Here's how the part is built. I have some questions about the finished solid (model axes, mm). Face numbers are marked on the shaded views. Round coordinates to 2 decimals unless told otherwise and drop trailing zeros. Order: outer loops, then holes, each group sorted by start corner. A loop starts at its lowest first (then second) coordinate and runs counter-clockwise, first axis right, second up.
```python
from build123d import *

# Parameters (mm, degrees)
CUT_EXTRUDE1_DEPTH      = 13.00023
CUT_EXTRUDE1_DEPTH_BACK = 13.00023
SKETCH3_R               = 7.9375
CUT_EXTRUDE3_DEPTH      = 13.7


with BuildPart() as part:
    # Sketch1 → Revolve1 (revolve)
    with BuildSketch(Plane(origin=(0, 0, 0), x_dir=(1, 0, 0), z_dir=(0, 1, 0))):
        with BuildLine():
            Line((0, 12.00023), (0, -12.00023))
            ThreePointArc((0, -12.00023), (12.00023, 0), (0, 12.00023))
        make_face()
    revolve(axis=Axis((0, 0, -16.515997735), (0, 0, 1)))

    # Sketch2 → Cut-Extrude1 (cut, two sides)
    with BuildSketch(Plane(origin=(0, 0, 0), x_dir=(0, 0, -1), z_dir=(1, 0, 0))) as cut_extrude1_sk:
        with BuildLine():
            Line((-6.35, 10.182485947), (-6.35, -10.182485947))
            ThreePointArc((-6.35, -10.182485947), (-12.00023, 0), (-6.35, 10.182485947))
        make_face()
        with BuildLine():
            ThreePointArc((6.35, -10.182485947), (12.00023, 0), (6.35, 10.182485947))
            Line((6.35, 10.182485947), (6.35, -10.182485947))
        make_face()
    extrude(amount=CUT_EXTRUDE1_DEPTH, mode=Mode.SUBTRACT)
    extrude(cut_extrude1_sk.sketch, amount=-CUT_EXTRUDE1_DEPTH_BACK, mode=Mode.SUBTRACT)

    # Sketch3 → Cut-Extrude3 (cut, through all)
    with BuildSketch(Plane.XY.offset(6.35)):
        Circle(SKETCH3_R)
    extrude(amount=-CUT_EXTRUDE3_DEPTH, mode=Mode.SUBTRACT)


solid = part.part
```
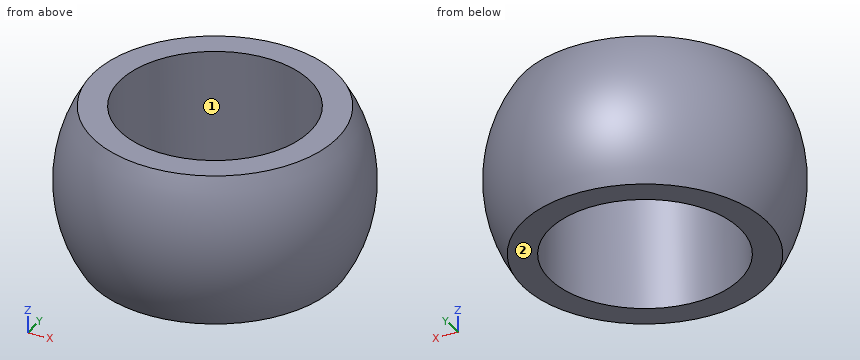
1) If we section it at C-C (z = 1.5): Write out the boundary of the cut face in (x, y) (1 decimal), plus the area to 3 significant figures.
2) I'm going to push flat-ended pins straight in: pin 1 (1.5 mm diameter, centred on x = 3.5, z = -0.5, fed in from +Y); pin 2 (1 mm diameter, centred on x = 8, z = -2.5, fed in from +Y); pin 3 (4 mm diameter, centred on x = -2, z = 3.5, fed in from -Y). Where does each tip first touch, or does it pass through?
3) We'd pull the mould along X, two halves only. Please class the marked faces 1 and 2: +X half, -X half, draft (parallel to the pull), parting line (faces both ways), or undercut.
4) I need wall thicknesses on line 1 (Y direction, x = -1.5, z = 3.25); line 2 (Y direction, x = 0, z = -2.5); line 3 (X direction, y = -4.5, z = -1.5). Which ranges of each line are inside material? Lowest first, please.
5) If we section it at D-D (y = 10.5): Write out the boundary of the cut face in (x, z).
6) If we section it at A-A (x = 0): Write out the boundary of the cut face in (y, z).
Solutions:
1. outline: circle Ø23.8 at (0, 0); hole circle Ø15.9 at (0, 0)
1. area: 247 mm2
2. pin 1: stops at y = 11.67
2. pin 2: stops at y = 9.05
2. pin 3: stops at y = -11.83
3. face 1: undercut
3. face 2: draft
4. line 1: y = -11.45 to -7.79, 7.79 to 11.45
4. line 2: y = -11.74 to -7.94, 7.94 to 11.74
4. line 3: x = -11.02 to -6.54, 6.54 to 11.02
5. outline: circle Ø11.62 at (0, 0)
6. outline: (-10.18, -6.35) - (-7.94, -6.35) - (-7.94, 6.35) - (-10.18, 6.35) arc R12 ccw to start; (7.94, -6.35) - (10.18, -6.35) arc R12 ccw to (10.18, 6.35) - (7.94, 6.35) - close
